Check sheet for the modelled part. Datum: model origin and axes. Units: mm. A direction names the side the tool comes from. Coordinates: 2 decimals unless noted, no trailing zeros. Loops run counter-clockwise (first coordinate to the right, second up) from the corner with the lowest first, then second, coordinate; pieces in that order, holes last. Notation, with made-up numbers: M 54,84 L 96,84 A14 ccw 96,108 Z; hole C 61,67 d10. An arc over 180 degrees is marked long. Write each question's results on one line, items separated by ' | '. Start each with the question number.
from build123d import *

# Parameters (mm, degrees)
SKETCH1_R      = 1.905
EXTRUDE1_DEPTH = 6.35


with BuildPart() as part:
    # Sketch1 → Extrude1 (new body)
    with BuildSketch(Plane(origin=(0, 0, 0), x_dir=(0, 0, -1), z_dir=(1, 0, 0))):
        Polygon((14.478, 0), (14.478, 6.35), (0, 6.35), (0, 12.7), (6.35, 12.7), (6.35, 38.1), (0, 38.1), (0, 50.8), (6.35, 50.8), (6.35, 76.2), (0, 76.2), (0, 85.852), (54.356, 85.852), (54.356, 76.2), (48.006, 76.2), (48.006, 50.8), (54.356, 50.8), (54.356, 38.1), (48.006, 38.1), (48.006, 12.7), (54.356, 12.7), (54.356, 6.35), (39.878, 6.35), (39.878, 0), align=None)
        with Locations((10.668, 72.39)):
            Circle(SKETCH1_R, mode=Mode.SUBTRACT)
        with Locations((43.688, 72.39)):
            Circle(SKETCH1_R, mode=Mode.SUBTRACT)
        with Locations((43.688, 46.99)):
            Circle(SKETCH1_R, mode=Mode.SUBTRACT)
        with Locations((10.668, 46.99)):
            Circle(SKETCH1_R, mode=Mode.SUBTRACT)
    extrude(amount=EXTRUDE1_DEPTH)


solid = part.part
Item 1: Section check A-A (y = 72.39). Record the cut outline in (x, z), plus the area to 3 significant figures.
Item 2: Section check D-D (y = 17). Record the cut outline in (x, z).
Item 3: Section check C-C (y = 46.99). Record the cut outline in (x, z), plus the area to 3 significant figures.
Item 4: Depth check by flat-ended pin: P1, Ø1.9, axis at x = 2, y = 62, coming from the -Z side; P2, Ø4, axis at y = 48, z = -40, coming from the -X side; P3, Ø3, axis at x = 3, z = -51.5, coming from the -Y side; P4, Ø3, axis at x = 3.5, y = 65.5, coming from the +Z side. Enter the tip coordinate at first touch or a pass-through.
Item 5: Release check for a two-part mould opening along Y. For faces 6 (the face through (3, 6.35, -7)), 7 (the face through (3, 44, 0)), 8 (the face through (3.13, 70.53, -10.26)) record: +Y half, -Y half, draft (parallel to the pull), parting line (faces both ways), or undercut.
Item 6: Thickness scan on line 1 (Z direction, x = 2.5, y = 72.39); line 2 (Y direction, x = 4, z = -49.5); line 3 (Z direction, x = 0.5, y = 46). Record the ranges inside material, lowest first.
Item 7: Section check B-B (x = 3.75). Record the cut outline in (y, z) (3 decimals).
Item 8: Tool access check on faces 1 (the face through (3, 3, -39.878)), 2 (the face through (3, 50.8, -51)), 3 (the face through (3, 25, -6.35)), 4 (the face through (3, 3, -14.478)), 5 (the face through (3, 10, -54.356)). Record the directions out of +Z, -Z, +X, -X, +Y, -Y that give a thin tool (end or side, any length) a straight path to the whole face; none if there is none.
Computed values:
1) outline: M 0,-48.01 L 6.35,-48.01 L 6.35,-45.59 L 0,-45.59 Z; M 0,-41.78 L 6.35,-41.78 L 6.35,-12.57 L 0,-12.57 Z; M 0,-8.76 L 6.35,-8.76 L 6.35,-6.35 L 0,-6.35 Z | area: 216 mm²
2) outline: M 0,-48.01 L 6.35,-48.01 L 6.35,-6.35 L 0,-6.35 Z
3) outline: M 0,-54.36 L 6.35,-54.36 L 6.35,-45.59 L 0,-45.59 Z; M 0,-41.78 L 6.35,-41.78 L 6.35,-12.57 L 0,-12.57 Z; M 0,-8.76 L 6.35,-8.76 L 6.35,0 L 0,0 Z | area: 297 mm²
4) P1: stops at z = -48.01 | P2: stops at x = 0 | P3: stops at y = 6.35 | P4: stops at z = -6.35
5) face 6: -Y half | face 7: draft | face 8: undercut
6) line 1: z = -48.01 to -45.59, -41.78 to -12.57, -8.76 to -6.35 | line 2: y = 6.35 to 12.7, 38.1 to 50.8, 76.2 to 85.85 | line 3: z = -54.36 to -45.32, -42.06 to -12.3, -9.04 to 0
7) outline: M 0,-39.878 L 6.35,-39.878 L 6.35,-54.356 L 12.7,-54.356 L 12.7,-48.006 L 38.1,-48.006 L 38.1,-54.356 L 50.8,-54.356 L 50.8,-48.006 L 76.2,-48.006 L 76.2,-54.356 L 85.852,-54.356 L 85.852,0 L 76.2,0 L 76.2,-6.35 L 50.8,-6.35 L 50.8,0 L 38.1,0 L 38.1,-6.35 L 12.7,-6.35 L 12.7,0 L 6.35,0 L 6.35,-14.478 L 0,-14.478 Z; hole C 46.99,-43.688 d3.81; hole C 46.99,-10.668 d3.81; hole C 72.39,-43.688 d3.81; hole C 72.39,-10.668 d3.81
8) face 1: -Z, +X, -X, -Y | face 2: -Z, +X, -X | face 3: +Z, +X, -X | face 4: +Z, +X, -X, -Y | face 5: -Z, +X, -X, +Y, -Y
